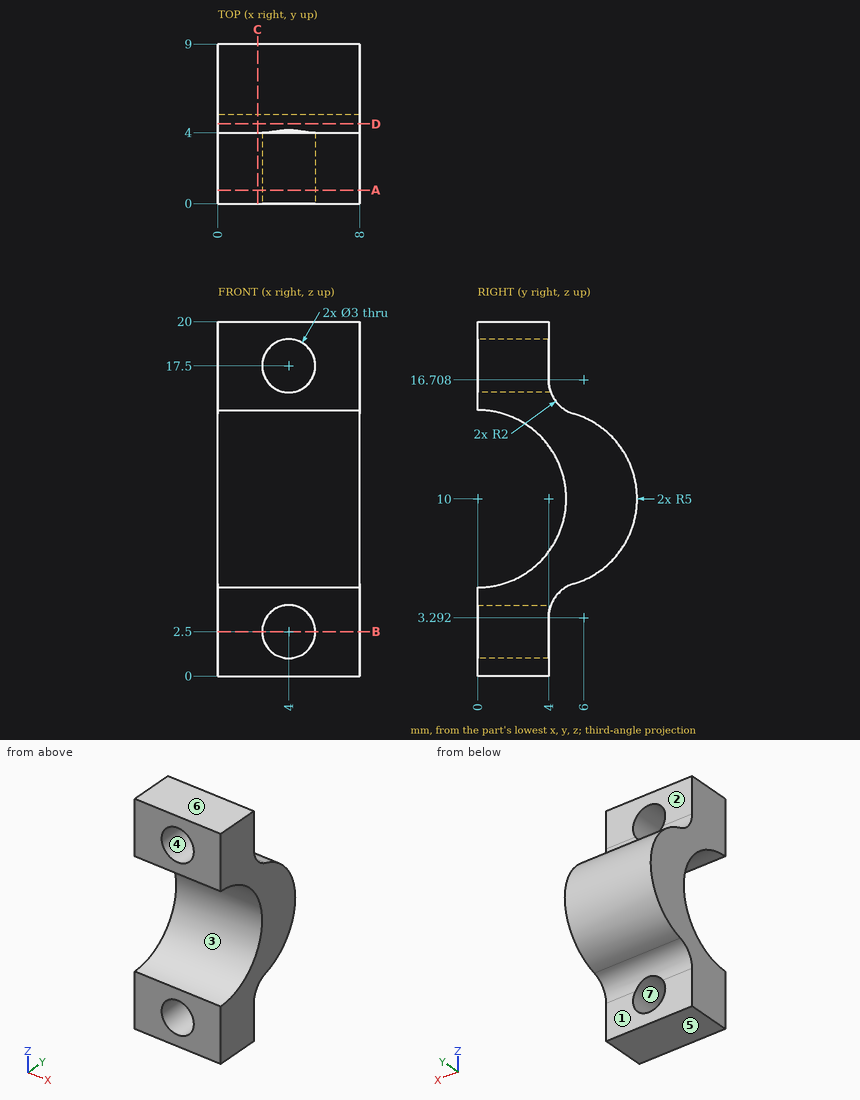
Could you check a few things on this drawing? It's one solid part, dimensions in mm from its lowest x, y, z. A direction names the side the tool comes from. Round coordinates to 2 decimals unless told otherwise and drop trailing zeros. Loops run counter-clockwise (first coordinate to the right, second up) from the corner with the lowest first, then second, coordinate; pieces in that order, holes last. Notation, with made-up numbers: (-9.75, -15) -> (43.25, -15) arc R10 cw to (43.25, -6) -> close; hole circle Ø5 at (53.5, 58). An arc over 180 degrees is marked (long way). One line per item, written item: value. Start each with the question number.
1. If we section it at B-B, the plane z = 2.5: Write out the boundary of the cut face in (x, y).
2. If we section it at C-C, the plane x = 2.25: Write out the boundary of the cut face in (y, z).
3. For pin 1 (1 mm diameter, centred on x = 5, z = 18.5, fed in from +Y); pin 2 (1 mm diameter, centred on x = 6.5, y = 7.5, fed in from +Z); pin 3 (1.5 mm diameter, centred on x = 5, z = 8.5, fed in from +Y), each with a flat end and sliding along its axis, tell me the tip position at first contact or that it passes through.
4. If we mould it in two halves opening along Z, with no side actions, what happens to the marked faces 4, 5, 6 and 7? For each: pulls with the +Z half, pulls with the -Z half, needs draft (parallel to the pull), parting line crosses it, or undercut.
5. For the marked faces 1, 2 and 3, which set-ups out of +Z, -Z, +X, -X, +Y, -Y let a thin tool reach every point of the face, with its end or its side?
6. If we section it at D-D, the plane y = 4.5: Write out the boundary of the cut face in (x, z) (1 decimal).
7. If I drill on probe 1 along X at (y, z) = (1.65, 17.5); probe 2 along Z at (x, y) = (5.25, 1.5); probe 3 along Z at (x, y) = (7.25, 3.75), over which ranges is the centre line in solid material (lowest first)?
8. If we section it at A-A, the plane y = 0.75: Write out the boundary of the cut face in (x, z).
Calculated:
1. outline: (0, 0) -> (2.5, 0) -> (2.5, 4) -> (0, 4) -> close; (5.5, 0) -> (8, 0) -> (8, 4) -> (5.5, 4) -> close
2. outline: (0, 0) -> (4, 0) -> (4, 3.29) arc R2 cw to (5.43, 5.21) arc R5 ccw to (5.43, 14.79) arc R2 cw to (4, 16.71) -> (4, 20) -> (0, 20) -> (0, 15) arc R5 cw to (0, 5) -> close
3. pin 1: stops at y = 4
3. pin 2: stops at z = 14
3. pin 3: stops at y = 8.94
4. face 4: undercut
4. face 5: pulls with the -Z half
4. face 6: pulls with the +Z half
4. face 7: undercut
5. face 1: -Z, +X, -X, +Y
5. face 2: +Z, +X, -X, +Y
5. face 3: +X, -X, -Y
6. outline: (0, 4.6) -> (8, 4.6) -> (8, 7.8) -> (0, 7.8) -> close; (0, 12.2) -> (8, 12.2) -> (8, 15.4) -> (0, 15.4) -> close
7. probe 1: x = 0 to 2.5, 5.5 to 8
7. probe 2: z = 0 to 1.67, 3.33 to 5.23, 14.77 to 16.67, 18.33 to 20
7. probe 3: z = 0 to 6.69, 13.31 to 20
8. outline: (0, 0) -> (8, 0) -> (8, 5.06) -> (0, 5.06) -> close; (0, 14.94) -> (8, 14.94) -> (8, 20) -> (0, 20) -> close; hole circle Ø3 at (4, 2.5); hole circle Ø3 at (4, 17.5)
